Geometry: final body of the model. Coordinates: model frame, mm. A direction names the side the tool comes from. Round coordinates to 2 decimals unless told otherwise and drop trailing zeros. Loops run counter-clockwise (first coordinate to the right, second up) from the corner with the lowest first, then second, coordinate; pieces in that order, holes last. Notation, with made-up numbers: (53, 88.25) -> (66, 88.25) arc R33 ccw to (66, 120.25) -> close; hole circle Ø9 at (61.25, -23.5). An arc over 180 degrees is marked (long way). Answer in a Markdown table with one row per item.
```python
from build123d import *

# Parameters (mm, degrees)
SKETCH2_R                   = 4
BOSS_EXTRUDE1_DEPTH         = 9.525
TAP_DRILL_FOR_M3X0_5_TAP1_D = 2.5
SKETCH7_W                   = 42.3
SKETCH7_H                   = 25.4
BOSS_EXTRUDE2_DEPTH         = 9.525
F_1_4_CLEARANCE_HOLE1_D     = 6.7564


with BuildPart() as part:
    # Sketch2 → Boss-Extrude1 (new body)
    # profile 1 of 6: a face of its own
    with BuildSketch(Plane(origin=(0, 0, 0), x_dir=(1, 0, 0), z_dir=(0, 1, 0))):
        Polygon((20, 0), (0, 0), (0, -39.537633496), (0, -58.85), (20, -58.85), (20, -39.537633496), align=None)
        with Locations(Location((10, -27.7, 0), (0, 0, 90))):
            Circle(SKETCH2_R, mode=Mode.SUBTRACT)
    # profile 2 of 6: a face of its own
    with BuildSketch(Plane(origin=(0, 0, 0), x_dir=(1, 0, 0), z_dir=(0, 1, 0))):
        Polygon((0, -58.85), (0, -39.537633496), (-11.15, -58.85), align=None)
    # profile 3 of 6: a face of its own
    with BuildSketch(Plane(origin=(0, 0, 0), x_dir=(1, 0, 0), z_dir=(0, 1, 0))):
        Polygon((31.15, -58.85), (20, -39.537633496), (20, -58.85), align=None)
    # profile 4 of 6: a face of its own
    with BuildSketch(Plane(origin=(0, 0, 0), x_dir=(1, 0, 0), z_dir=(0, 1, 0))):
        with BuildLine():
            Line((0, -72.5), (0, -58.85))
            Line((0, -58.85), (-11.15, -58.85))
            Line((-11.15, -58.85), (-11.15, -101.15))
            Line((-11.15, -101.15), (31.15, -101.15))
            Line((31.15, -101.15), (31.15, -58.85))
            Line((31.15, -58.85), (20, -58.85))
            Line((20, -58.85), (20, -72.5))
            ThreePointArc((20, -72.5), (21.858541226, -76.047152925), (22.5, -80))
            ThreePointArc((22.5, -80), (21.858541226, -83.952847075), (20, -87.5))
            Line((20, -87.5), (20, -100))
            Line((20, -100), (0, -100))
            Line((0, -100), (0, -87.5))
            ThreePointArc((0, -87.5), (-2.5, -80), (0, -72.5))
        make_face()
    # profile 5 of 6: a face of its own
    with BuildSketch(Plane(origin=(0, 0, 0), x_dir=(1, 0, 0), z_dir=(0, 1, 0))):
        with BuildLine():
            Line((20, -58.85), (0, -58.85))
            Line((0, -58.85), (0, -72.5))
            ThreePointArc((0, -72.5), (10, -67.5), (20, -72.5))
            Line((20, -72.5), (20, -58.85))
        make_face()
    # profile 6 of 6: a face of its own
    with BuildSketch(Plane(origin=(0, 0, 0), x_dir=(1, 0, 0), z_dir=(0, 1, 0))):
        with BuildLine():
            ThreePointArc((20, -87.5), (10, -92.5), (0, -87.5))
            Line((0, -87.5), (0, -100))
            Line((0, -100), (20, -100))
            Line((20, -100), (20, -87.5))
        make_face()
    extrude(amount=BOSS_EXTRUDE1_DEPTH)

    # Tap Drill for M3x0.5 Tap1 (through all)
    with Locations(Plane(origin=(0, 9.525, 0), x_dir=(1, 0, 0), z_dir=(0, 1, 0))):
        with Locations((-5.5, -64.5), (25.5, -64.5), (25.5, -95.5), (-5.5, -95.5)):
            Hole(TAP_DRILL_FOR_M3X0_5_TAP1_D / 2)

    # Sketch7 → Boss-Extrude2 (add)
    with BuildSketch(Plane(origin=(0, 9.525, 0), x_dir=(1, 0, 0), z_dir=(0, 1, 0))):
        with Locations((10, -113.85)):
            Rectangle(SKETCH7_W, SKETCH7_H)
    extrude(amount=-BOSS_EXTRUDE2_DEPTH)

    # 1/4 Clearance Hole1 (through all)
    with Locations(Plane(origin=(0, 9.525, 0), x_dir=(1, 0, 0), z_dir=(0, 1, 0))):
        with Locations((-2, -113.85), (22, -113.85)):
            Hole(F_1_4_CLEARANCE_HOLE1_D / 2)


solid = part.part
```
Item 1: Section query C-C, the plane y = 6. State how many separate pieces and enclosed holes the cut face has, and give its area (3 significant figures).
Ans:
| item | result |
|---|---|
| separate pieces | 1 |
| enclosed holes | 8 |
| area | 3,620 mm2 |
Item 2: First-contact query: P1, Ø2, axis at x = 25.5, z = 64.5, coming from the +Y side; P2, Ø3, axis at y = 2.5, z = 27, coming from the +X side; P3, Ø2, axis at x = 26.5, y = 6, coming from the -Z side. Flat tips, straight axial feed; report the tip coordinate or a pass-through.
Ans:
| item | result |
|---|---|
| P1 | through |
| P2 | x = 20 |
| P3 | z = 49.06 |
Item 3: Section query A-A, the plane z = 80. Output: boundary loops of the cut face in (x, y) (3 decimals), and give its area (3 significant figures).
Ans:
| item | result |
|---|---|
| outline | (-11.15, 0) -> (-2.5, 0) -> (-2.5, 9.525) -> (-11.15, 9.525) -> close; (22.5, 0) -> (31.15, 0) -> (31.15, 9.525) -> (22.5, 9.525) -> close |
| area | 165 mm2 |
Item 4: Ray query, L1, parallel to X at y = 7.75, z = 95.5; L2, parallel to Z at x = 10, y = 3.5; L3, parallel to X at y = 3.5, z = 87.5. Return the intervals inside material, ascending.
Ans:
| item | result |
|---|---|
| L1 | -11.15 to -6.75, -4.25 to 24.25, 26.75 to 31.15 |
| L2 | 0 to 23.7, 31.7 to 67.5, 92.5 to 126.55 |
| L3 | -11.15 to 0, 20 to 31.15 |
Item 5: Set-up query: faces 4 (the cylindrical face through (20.441, 4.696, 116.847)), 5 (the flat face through (0, 5, 19)), 6 (the flat face through (20, 5, 20)). Return all of +Z, -Z, +X, -X, +Y, -Y with unobstructed straight access to the full face (end or side cutting, diameter ignored); none if empty.
Ans:
| item | result |
|---|---|
| face 4 | +Y, -Y |
| face 5 | -Z, -X, +Y, -Y |
| face 6 | -Z, +X, +Y, -Y |
Item 6: Mould query, pull axis X, two halves, no side actions, for faces 1 (the flat face through (31.15, 5, 93)), 2 (the cylindrical face through (-5.34, 4.7, 94.26)), 3 (the flat face through (10, 0, 62)). Classes: released by +X, released by -X, zero draft, split by the parting line, or undercut.
Ans:
| item | result |
|---|---|
| face 1 | released by +X |
| face 2 | undercut |
| face 3 | zero draft |
Item 7: Section query B-B, the plane x = 17.5. Output: boundary loops of the cut face in (y, z) (3 decimals).
Ans:
| item | result |
|---|---|
| outline | (0, 0) -> (9.525, 0) -> (9.525, 70) -> (0, 70) -> close; (0, 90) -> (9.525, 90) -> (9.525, 126.55) -> (0, 126.55) -> close |
Item 8: Section query D-D, the plane z = 113.85. Output: boundary loops of the cut face in (x, y) (3 decimals), and give its area (3 significant figures).
Ans:
| item | result |
|---|---|
| outline | (-11.15, 0) -> (-5.378, 0) -> (-5.378, 9.525) -> (-11.15, 9.525) -> close; (1.378, 0) -> (18.622, 0) -> (18.622, 9.525) -> (1.378, 9.525) -> close; (25.378, 0) -> (31.15, 0) -> (31.15, 9.525) -> (25.378, 9.525) -> close |
| area | 274 mm2 |
